Verification items for the finished model (mm, model axes). Face numbers are marked on the shaded views. A direction names the side the tool comes from. Give positions to 0.01 mm unless a question says otherwise; leave off trailing zeros. Order: outer loops, then holes, each group sorted by start corner. A loop starts at its lowest first (then second) coordinate and runs counter-clockwise, first axis right, second up. Notation, with made-up numbers: (18, -9) - (71, -9) arc R19 cw to (71, 22) - close; hole circle Ø3 at (9, -26.75). An arc over 180 degrees is marked (long way). Answer as a JSON object with one key per item and string values.
```python
from build123d import *

# Parameters (mm, degrees)
SKETCH2_R                = 30
BOSS_EXTRUDE4_DEPTH      = 2.54
BOSS_EXTRUDE4_DEPTH_BACK = 12.7
SKETCH1_R                = 62.75
CUT_EXTRUDE5_DEPTH       = 31
CUT_EXTRUDE5_DEPTH_BACK  = 31
CUT_EXTRUDE6_DEPTH       = 31.0000001
CUT_EXTRUDE6_DEPTH_BACK  = 31.0000001
SKETCH12_R               = 17.47
BOSS_EXTRUDE7_DEPTH      = 30
BOSS_EXTRUDE7_DEPTH_BACK = 20
SKETCH20_R               = 15.9
CUT_EXTRUDE8_DEPTH       = 51.0000001
CHAMFER1_SIZE            = 0.75
FILLET1_R                = 0.7
LPATTERN1_COUNT          = 5
LPATTERN1_PITCH          = 4


with BuildPart() as part:
    # Sketch2 → Boss-Extrude4 (new body, two sides)
    with BuildSketch(Plane.XY.offset(63.5)) as boss_extrude4_sk:
        Circle(SKETCH2_R)
    extrude(amount=BOSS_EXTRUDE4_DEPTH)
    extrude(boss_extrude4_sk.sketch, amount=-BOSS_EXTRUDE4_DEPTH_BACK)

    # Sketch1 → Cut-Extrude5 (cut, two sides)
    with BuildSketch(Plane(origin=(0, 0, 0), x_dir=(1, 0, 0), z_dir=(0, 1, 0))) as cut_extrude5_sk:
        Circle(SKETCH1_R)
    extrude(amount=CUT_EXTRUDE5_DEPTH, mode=Mode.SUBTRACT)
    extrude(cut_extrude5_sk.sketch, amount=-CUT_EXTRUDE5_DEPTH_BACK, mode=Mode.SUBTRACT)

    # Sketch11 → Cut-Extrude6 (cut, two sides)
    with BuildSketch(Plane(origin=(0, 0, 0), x_dir=(1, 0, 0), z_dir=(0, 1, 0))) as cut_extrude6_sk:
        with BuildLine():
            Line((31.285011062, -58.15951928), (31.285011062, -70.975470201))
            Line((31.285011062, -70.975470201), (-30.859364653, -70.975470201))
            Line((-30.859364653, -70.975470201), (-30.859364653, -58.386481425))
            ThreePointArc((-30.859364653, -58.386481425), (0.241188039, -66.039559571), (31.285011062, -58.15951928))
        make_face()
    extrude(amount=CUT_EXTRUDE6_DEPTH, mode=Mode.SUBTRACT)
    extrude(cut_extrude6_sk.sketch, amount=-CUT_EXTRUDE6_DEPTH_BACK, mode=Mode.SUBTRACT)

    # Sketch12 → Boss-Extrude7 (add, two sides)
    with BuildSketch(Plane.XY.offset(63.5)) as boss_extrude7_sk:
        Circle(SKETCH12_R)
    extrude(amount=BOSS_EXTRUDE7_DEPTH)
    extrude(boss_extrude7_sk.sketch, amount=-BOSS_EXTRUDE7_DEPTH_BACK)

    # Sketch20 → Cut-Extrude8 (cut, through all)
    with BuildSketch(Plane.XY.offset(93.5)):
        Circle(SKETCH20_R)
    extrude(amount=-CUT_EXTRUDE8_DEPTH, mode=Mode.SUBTRACT)

    # Chamfer1
    chamfer1_edges = [part.edges().sort_by_distance(p)[0] for p in [
        (-15.9, 0, 93.5),
    ]]
    chamfer(chamfer1_edges, length=CHAMFER1_SIZE)

    # Fillet1
    fillet1_edges = [part.edges().sort_by_distance(p)[0] for p in [
        (-17.47, 0, 43.5),
        (-15.9, 0, 43.5),
    ]]
    fillet(fillet1_edges, radius=FILLET1_R)

    # Sketch23 → Revolve1 (revolve)
    with BuildSketch(Plane(origin=(0, 0, 0), x_dir=(0, 0, -1), z_dir=(1, 0, 0))):
        Polygon((-92.75, 15.9), (-88.75, 15.9), (-88.75, 15.4), align=None)
    revolve1 = revolve(axis=Axis((0, 0, 93.5), (0, 0, -1)))

    # LPattern1: Revolve1 ×5
    with Locations(*[(0, 0, -i * LPATTERN1_PITCH) for i in range(1, LPATTERN1_COUNT)]):
        add(revolve1)


solid = part.part
```
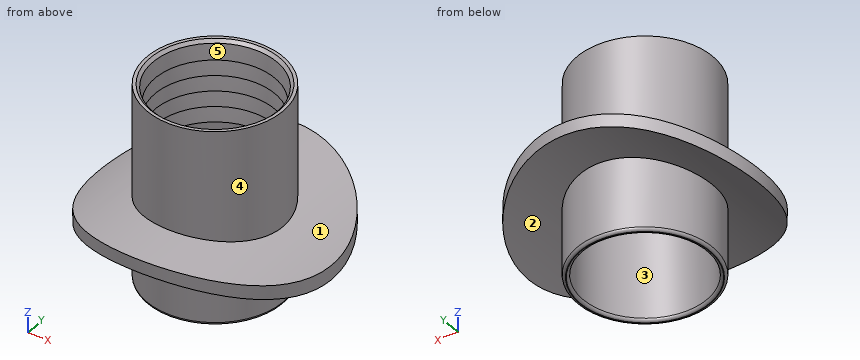
(1) Section check A-A (z = 51). Record the cut outline in (x, y).
Computed values:
{"outline": "circle Ø34.94 at (0, 0); hole circle Ø31.8 at (0, 0)"}
(2) Access from +Z, -Z, +X, -X, +Y, -Y to the whole of each face (thin tool, end or side, straight path). Record for the marked faces 1 and 2.
Computed values:
{"face 1": "+Z", "face 2": "-Z"}
(3) Section check B-B (y = 23). Record the cut outline in (x, z).
Computed values:
{"outline": "(-19.26, 59.72) arc R62.75 cw to (19.26, 59.72) - (19.26, 63.17) arc R66.04 ccw to (-19.26, 63.17) - close"}
(4) Gauge pin test, flat ends, axial feed: pin 1 Ø1.5 at (y, z) = (-9, 81) entering from -X; pin 2 Ø3 at (x, z) = (11.5, 54.5) entering from +Y; pin 3 Ø12 at (x, z) = (-20.5, 83.5) entering from -Y. Record the tip position at first contact, or that the pin passes through.
Computed values:
{"pin 1": "stops at x = -15.4", "pin 2": "stops at y = 14.32", "pin 3": "stops at y = -9.74"}
(5) Release check for a two-part mould opening along Y. For the marked faces 3, 4 and 5 record: pulls with the +Y half, pulls with the -Y half, needs draft (parallel to the pull), parting line crosses it, or undercut.
Computed values:
{"face 3": "undercut", "face 4": "parting line crosses it", "face 5": "undercut"}
(6) Material ranges on line 1 along Y through (x, z) = (0, 57); line 2 along Y through (x, z) = (0, 64.25); line 3 along X through (y, z) = (14.5, 80), recorded low to high. Write a range as [from, to].
Computed values:
{"line 1": "y = [-17.47, -15.9], [15.9, 17.47]", "line 2": "y = [-30, -15.9], [15.9, 30]", "line 3": "x = [-9.74, -6.29], [6.29, 9.74]"}
(7) Section check C-C (x = -23). Record the cut outline in (y, z).
Computed values:
{"outline": "(-19.26, 58.38) - (19.26, 58.38) - (19.26, 61.91) - (-19.26, 61.91) - close"}
(8) Section check D-D (z = 90.5). Record the cut outline in (x, y), then the cut area to 3 significant figures.
Computed values:
{"outline": "circle Ø34.94 at (0, 0); hole circle Ø31.24 at (0, 0)", "area": "192 mm²"}
